Source: CAD feature listing. Evaluate the final solid. Frame: model axes, mm. Round coordinates to 2 decimals unless told otherwise and drop trailing zeros. Loops run counter-clockwise (first coordinate to the right, second up) from the corner with the lowest first, then second, coordinate; pieces in that order, holes last.
Item 1: Section query C-C on x = 6. Return loops of the section in (y, z).
Item 2: Ray query, L1, parallel to X at y = 0.85, z = 32.5; L2, parallel to Z at x = -43.5, y = 1.6; L3, parallel to Z at x = 4, y = -0.2. Return the intervals inside material, ascending.
Item 3: Section query D-D on x = -39.5. Return loops of the section in (y, z), then the cut area to 3 significant figures.
Item 4: Section query A-A on x = 43.5. Return loops of the section in (y, z), then the cut area to 3 significant figures.
Item 5: Section query B-B on z = 4. Return loops of the section in (x, y).
Item 6: First-contact query: P1, Ø2.5, axis at x = 8, y = -2, coming from the +Z side; P2, Ø12, axis at x = 5, z = -18, coming from the -Y side; P3, Ø0.8, axis at y = -2, z = -0.5, coming from the +X side; P4, Ø2.5, axis at x = -43.5, z = 32.5, coming from the +Y side. Flat tips, straight axial feed; report the tip coordinate or a pass-through.
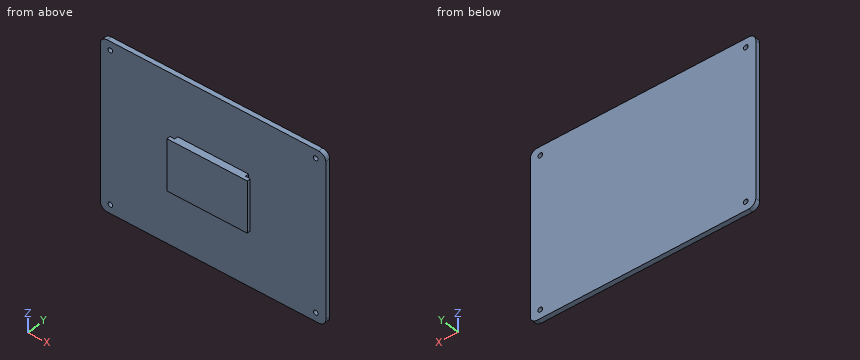
```python
from build123d import *

# Parameters (mm, degrees)
EXTRUDE_1_DEPTH          = 2
SKETCH_3_R               = 1
CUT_EXTRUDE_1_DEPTH      = 3
CUT_EXTRUDE_1_DEPTH_BACK = 13
SKETCH_4_W               = 34
SKETCH_4_H               = 22
EXTRUDE_3_DEPTH          = 3
SKETCH_5_W               = 2
SKETCH_5_H               = 22
CUT_EXTRUDE_3_DEPTH      = 1.5


with BuildPart() as part:
    # Эскиз1 → Бобышка-Вытянуть1 (new body)
    with BuildSketch(Plane(origin=(0, 0, 0), x_dir=(1, 0, 0), z_dir=(0, 1, 0))):
        with BuildLine():
            Line((-47.75, -33.25), (-47.75, 33.25))
            ThreePointArc((-47.75, 33.25), (-46.871320344, 35.371320344), (-44.75, 36.25))
            Line((-44.75, 36.25), (44.75, 36.25))
            ThreePointArc((44.75, 36.25), (46.871320344, 35.371320344), (47.75, 33.25))
            Line((47.75, 33.25), (47.75, -33.25))
            ThreePointArc((47.75, -33.25), (46.871320344, -35.371320344), (44.75, -36.25))
            Line((44.75, -36.25), (-44.75, -36.25))
            ThreePointArc((-44.75, -36.25), (-46.871320344, -35.371320344), (-47.75, -33.25))
        make_face()
    extrude(amount=EXTRUDE_1_DEPTH)

    # Эскиз3 → Вырез-Вытянуть1 (cut, two sides)
    with BuildSketch(Plane(origin=(0, 5, 0), x_dir=(1, 0, 0), z_dir=(0, 1, 0))) as cut_extrude_1_sk:
        with Locations((-43.5, 32.5)):
            Circle(SKETCH_3_R)
        with Locations((-43.5, -32.5)):
            Circle(SKETCH_3_R)
        with Locations((43.5, -32.5)):
            Circle(SKETCH_3_R)
        with Locations((43.5, 32.5)):
            Circle(SKETCH_3_R)
    extrude(amount=CUT_EXTRUDE_1_DEPTH, mode=Mode.SUBTRACT)
    extrude(cut_extrude_1_sk.sketch, amount=-CUT_EXTRUDE_1_DEPTH_BACK, mode=Mode.SUBTRACT)

    # Эскиз4 → Бобышка-Вытянуть3 (add)
    with BuildSketch(Plane.XZ):
        Rectangle(SKETCH_4_W, SKETCH_4_H)
    extrude(amount=EXTRUDE_3_DEPTH)

    # Эскиз5 → Вырез-Вытянуть3 (cut)
    with BuildSketch(Plane.XZ):
        with Locations((-16, 0)):
            Rectangle(SKETCH_5_W, SKETCH_5_H)
        with Locations((16, 0)):
            Rectangle(SKETCH_5_W, SKETCH_5_H)
    extrude(amount=CUT_EXTRUDE_3_DEPTH, mode=Mode.SUBTRACT)


solid = part.part
```
Data:
1. outline: (-3, -11) - (0, -11) - (0, -36.25) - (2, -36.25) - (2, 36.25) - (0, 36.25) - (0, 11) - (-3, 11) - close
2. L1: x = -47.75 to -44.5, -42.5 to 42.5, 44.5 to 47.75
2. L2: z = -36.25 to -33.5, -31.5 to 31.5, 33.5 to 36.25
2. L3: z = -11 to 11
3. outline: (0, -36.25) - (2, -36.25) - (2, 36.25) - (0, 36.25) - close
3. area: 145 mm2
4. outline: (0, -36.25) - (2, -36.25) - (2, -33.5) - (0, -33.5) - close; (0, -31.5) - (2, -31.5) - (2, 31.5) - (0, 31.5) - close; (0, 33.5) - (2, 33.5) - (2, 36.25) - (0, 36.25) - close
4. area: 137 mm2
5. outline: (-47.75, 0) - (-15, 0) - (-15, -1.5) - (-17, -1.5) - (-17, -3) - (17, -3) - (17, -1.5) - (15, -1.5) - (15, 0) - (47.75, 0) - (47.75, 2) - (-47.75, 2) - close
6. P1: stops at z = 11
6. P2: stops at y = 0
6. P3: stops at x = 17
6. P4: stops at y = 2
